The listing builds one solid part. Answer for the finished solid, in the listing's coordinates (mm). A direction names the side the tool comes from. Round coordinates to 2 decimals unless told otherwise and drop trailing zeros. Order: outer loops, then holes, each group sorted by start corner. A loop starts at its lowest first (then second) coordinate and runs counter-clockwise, first axis right, second up. Notation, with made-up numbers: (12, 48) -> (44, 48) arc R20 ccw to (44, 70) -> close; hole circle Ø10 at (8.25, -23.75). An arc over 180 degrees is marked (long way). Return JSON: item names as keys, results as strings. Group by question number.
(1) Consider line 1 (Y direction, x = 362, z = 2.5); line 2 (Y direction, x = 28, z = 27.5); line 3 (Y direction, x = 191, z = 38.5). Determine where each line is inside the solid, lowest interval first. Write a range as [from, to].
(2) The part is cut by section C-C (x = 374.5). Determine the outline of the cut face in (y, z), plus the area to 3 significant figures.
(3) Determine the mould class of faces 1 (the face through (364, 251, 40)), 2 (the face through (197, 480, 2)), 3 (the face through (197, 500, 20)) for opening direction Y: +Y half, -Y half, draft (parallel to the pull), parting line (faces both ways), or undercut.
(4) The part is cut by section D-D (y = 379). Determine the outline of the cut face in (x, z), plus the area to 3 significant figures.
(5) Which of the six approach directions +Z, -Z, +X, -X, +Y, -Y give full straight-line access (tool end or side, diameter ignored) to faces 4 (the face through (0, 478, 39)), 5 (the face through (197, 20, 38)), 6 (the face through (183, 460, 20))?
(6) This flat-tipped pin is pushed along its axis until it touches: pin 1 (8 mm diameter, centred on y = 75, z = 25, fed in from -X). Where does it stop, or does it pass through?
(7) The part is cut by section B-B (z = 7.5). Determine the outline of the cut face in (x, y), plus the area to 3 significant figures.
(8) The part is cut by section A-A (x = 71). Determine the outline of the cut face in (y, z).
from build123d import *

# Parameters (mm, degrees)
BOSS_EXTRUDE1_DEPTH = 40
SKETCH3_W           = 36
SKETCH3_H           = 36
CUT_EXTRUDE1_DEPTH  = 448
SKETCH4_W           = 36
SKETCH4_H           = 36
CUT_EXTRUDE2_DEPTH  = 448


with BuildPart() as part:
    # Sketch2 → Boss-Extrude1 (new body)
    with BuildSketch(Plane.XY):
        Polygon((0, 0), (0, 40), (360, 40), (360, 460), (0, 460), (0, 500), (400, 500), (400, 0), align=None)
    extrude(amount=BOSS_EXTRUDE1_DEPTH)

    # Sketch3 → Cut-Extrude1 (cut)
    with BuildSketch(Plane.ZY):
        with Locations((20, 480)):
            Rectangle(SKETCH3_W, SKETCH3_H)
    extrude(amount=-CUT_EXTRUDE1_DEPTH, mode=Mode.SUBTRACT)

    # Sketch4 → Cut-Extrude2 (cut)
    with BuildSketch(Plane.ZY):
        with Locations((20, 20)):
            Rectangle(SKETCH4_W, SKETCH4_H)
    extrude(amount=-CUT_EXTRUDE2_DEPTH, mode=Mode.SUBTRACT)


solid = part.part
Answer below:
{
 "1": {"line 1": "y = [0, 2], [38, 462], [498, 500]", "line 2": "y = [0, 2], [38, 40], [460, 462], [498, 500]", "line 3": "y = [0, 40], [460, 500]"},
 "2": {"outline": "(0, 0) -> (500, 0) -> (500, 40) -> (0, 40) -> close; hole (2, 2) -> (38, 2) -> (38, 38) -> (2, 38) -> close; hole (462, 2) -> (498, 2) -> (498, 38) -> (462, 38) -> close", "area": "17,400 mm²"},
 "3": {"face 1": "draft", "face 2": "undercut", "face 3": "+Y half"},
 "4": {"outline": "(360, 0) -> (400, 0) -> (400, 40) -> (360, 40) -> close", "area": "1,600 mm²"},
 "5": {"face 4": "+Z, -Z, -X, +Y, -Y", "face 5": "+X, -X", "face 6": "+Z, -Z, -X"},
 "6": {"pin 1": "stops at x = 360"},
 "7": {"outline": "(0, 0) -> (400, 0) -> (400, 2) -> (0, 2) -> close; (0, 38) -> (400, 38) -> (400, 462) -> (0, 462) -> (0, 460) -> (360, 460) -> (360, 40) -> (0, 40) -> close; (0, 498) -> (400, 498) -> (400, 500) -> (0, 500) -> close", "area": "20,000 mm²"},
 "8": {"outline": "(0, 0) -> (40, 0) -> (40, 40) -> (0, 40) -> close; (460, 0) -> (500, 0) -> (500, 40) -> (460, 40) -> close; hole (2, 2) -> (38, 2) -> (38, 38) -> (2, 38) -> close; hole (462, 2) -> (498, 2) -> (498, 38) -> (462, 38) -> close"}
}
